```python
from build123d import *

# Parameters (mm, degrees)
SKETCH_1_W          = 32
SKETCH_1_H          = 10
SKETCH_1_R          = 1.5
EXTRUDE_1_DEPTH     = 0.5
OTHER_START         = -5
OTHER_1_DEPTH       = 10
OTHER_1_2_DEPTH     = 3.4999999
OTHER_START_2       = 1.5000001
OTHER_1_3_DEPTH     = 3.4999999
OTHER_START_3       = -1.5000001
OTHER_1_4_DEPTH     = 3.0000001
OTHER_START_4       = 5.910951377
OTHER_1_5_OUTLINE_R = 1.5
OTHER_1_5_DEPTH     = 0.5
FILLET_1_R          = 2


with BuildPart() as part:
    # Sketch 1 → Бобышка-Вытянуть1 (new body)
    with BuildSketch(Plane(origin=(0, 0, 0), x_dir=(1, 0, 0), z_dir=(0, 1, 0))):
        Rectangle(SKETCH_1_W, SKETCH_1_H)
        with Locations(Location((11, 0, 0), (0, 0, 270))):
            Circle(SKETCH_1_R, mode=Mode.SUBTRACT)
        with BuildLine():
            Line((-12, 1.5), (-5, 1.5))
            ThreePointArc((-5, 1.5), (-3.5, 0), (-5, -1.5))
            Line((-5, -1.5), (-12, -1.5))
            ThreePointArc((-12, -1.5), (-13.5, 0), (-12, 1.5))
        make_face(mode=Mode.SUBTRACT)
    extrude(amount=EXTRUDE_1_DEPTH)

    # Other 1: read off the stored shape, not the designer's step
    # Other 1 outline → Other 1 (cut)
    with BuildSketch(Plane.XY.offset(OTHER_START)):
        with BuildLine():
            Line((16, 0.5), (6.276976781, 0.5))
            ThreePointArc((6.276976781, 0.5), (5.910951377, 0.133974596), (5.410951377, 0))
            Line((5.410951377, 0), (16, 0))
            Line((16, 0), (16, 0.5))
        make_face()
    extrude(amount=OTHER_1_DEPTH, mode=Mode.SUBTRACT)

    # Other 1 2 outline → Other 1 2 (add)
    with BuildSketch(Plane.XY.offset(OTHER_START)):
        with BuildLine():
            Line((6.410951377, 1), (6.410951377, 10.410951377))
            Line((6.410951377, 10.410951377), (5.910951377, 10.410951377))
            Line((5.910951377, 10.410951377), (5.910951377, 1))
            ThreePointArc((5.910951377, 1), (5.764504768, 0.646446609), (5.410951377, 0.5))
            Line((5.410951377, 0.5), (6.276976781, 0.5))
            ThreePointArc((6.276976781, 0.5), (6.376877204, 0.741180955), (6.410951377, 1))
        make_face()
    extrude(amount=OTHER_1_2_DEPTH)

    # Other 1 3 outline → Other 1 3 (add)
    with BuildSketch(Plane.XY.offset(OTHER_START_2)):
        with BuildLine():
            Line((6.410951377, 1), (6.410951377, 10.410951377))
            Line((6.410951377, 10.410951377), (5.910951377, 10.410951377))
            Line((5.910951377, 10.410951377), (5.910951377, 1))
            ThreePointArc((5.910951377, 1), (5.764504768, 0.646446609), (5.410951377, 0.5))
            Line((5.410951377, 0.5), (6.276976781, 0.5))
            ThreePointArc((6.276976781, 0.5), (6.376877204, 0.741180955), (6.410951377, 1))
        make_face()
    extrude(amount=OTHER_1_3_DEPTH)

    # Other 1 4 outline → Other 1 4 (add)
    with BuildSketch(Plane.XY.offset(OTHER_START_3)):
        with BuildLine():
            Line((6.410951377, 1), (6.410951377, 10.410951377))
            Line((6.410951377, 10.410951377), (5.910951377, 10.410951377))
            Line((5.910951377, 10.410951377), (5.910951377, 1))
            ThreePointArc((5.910951377, 1), (5.764504768, 0.646446609), (5.410951377, 0.5))
            Line((5.410951377, 0.5), (6.276976781, 0.5))
            ThreePointArc((6.276976781, 0.5), (6.376877204, 0.741180955), (6.410951377, 1))
        make_face()
    extrude(amount=OTHER_1_4_DEPTH)

    # Other 1 5 outline → Other 1 5 (cut)
    with BuildSketch(Plane.YZ.offset(OTHER_START_4)):
        with Locations((5.410951377, 0)):
            Circle(OTHER_1_5_OUTLINE_R)
    extrude(amount=OTHER_1_5_DEPTH, mode=Mode.SUBTRACT)

    # Скругление1
    fillet_1_edges = [part.edges().sort_by_distance(p)[0] for p in [
        (6.160951377, 10.410951377, -5),
        (6.160951377, 10.410951377, 5),
        (-16, 0.25, 5),
        (-16, 0.25, -5),
    ]]
    fillet(fillet_1_edges, radius=FILLET_1_R)


solid = part.part
```
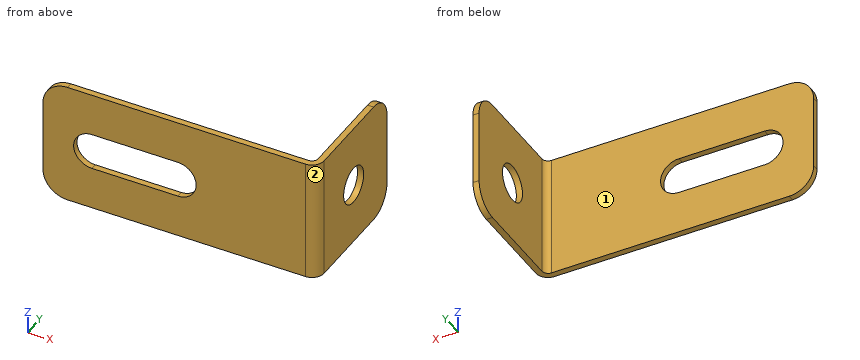
Part model, mm, in its own coordinate system. Face numbers are marked on the shaded views. A direction names the side the tool comes from. Give positions to 0.01 mm unless a question says otherwise; leave off trailing zeros. Order: outer loops, then holes, each group sorted by start corner. A loop starts at its lowest first (then second) coordinate and runs counter-clockwise, first axis right, second up. Notation, with made-up numbers: M 21,29.25 L 52,29.25 A12 ccw 52,45.25 Z; hole C -3,79 d7. An arc over 180 degrees is marked long. Use a Markdown table: item, result. Add a question column.
(1) Saw through at C-C, the plane z = 2.5. Give the cut face in (x, y).
(2) Saw through at D-D, the plane y = 5. Give the cut face in (x, z).
(3) Saw through at A-A, the plane z = 0. Give the cut face in (x, y).
(4) Probe line 1 along X through (y, z) = (7.75, 1); line 2 along Y through (x, z) = (4.75, 3). List the from-to ranges inside material, lowest first. Write a range as [from, to].
(5) Drop flat-ended pins along their axis: P1, Ø1.5, axis at x = -2.5, z = -4, coming from the +Y side; P2, Ø5, axis at y = 7, z = -0.5, coming from the -X side. Give the stop position or say it passes through.
(6) Saw through at B-B, the plane x = -9. Give the cut face in (y, z).
(7) 3-axis set-ups, long thin cutter, end or side, ignore diameter. For the marked faces 1 and 2: which of +Z, -Z, +X, -X, +Y, -Y reach the whole face in a straight line?
Answer key:
| question | item | result |
|---|---|---|
| 1 | outline | M -16,0 L 5.41,0 A1 ccw 6.41,1 L 6.41,10.41 L 5.91,10.41 L 5.91,1 A0.5 cw 5.41,0.5 L -16,0.5 Z |
| 2 | outline | M 5.91,-5 L 6.41,-5 L 6.41,-1.44 L 5.91,-1.44 Z; M 5.91,1.44 L 6.41,1.44 L 6.41,5 L 5.91,5 Z |
| 3 | outline | M -16,0 L -13.5,0 L -13.5,0.5 L -16,0.5 Z; M -3.5,0 L 5.41,0 A1 ccw 6.41,1 L 6.41,3.91 L 5.91,3.91 L 5.91,1 A0.5 cw 5.41,0.5 L -3.5,0.5 Z; M 5.91,6.91 L 6.41,6.91 L 6.41,10.41 L 5.91,10.41 Z |
| 4 | line 1 | [5.91, 6.41] |
| 4 | line 2 | [0, 0.5] |
| 5 | P1 | y = 0.5 |
| 5 | P2 | x = 5.91 |
| 6 | outline | M 0,-5 L 0.5,-5 L 0.5,-1.5 L 0,-1.5 Z; M 0,1.5 L 0.5,1.5 L 0.5,5 L 0,5 Z |
| 7 | face 1 | +Z, -Z, -X, +Y |
| 7 | face 2 | +Z, -Z, +X, -Y |
